```python
from build123d import *

# Parameters (mm, degrees)
PAD_DEPTH = 2.3


with BuildPart() as part:
    # Sketch → Pad (new body)
    with BuildSketch(Plane.XY):
        with BuildLine():
            Line((0, 0), (50, 0))
            Line((50, 0), (50, 30))
            Line((44.25, 30), (50, 30))
            Line((44.25, 30), (44.25, 23))
            ThreePointArc((39.75, 23), (42, 20.75), (44.25, 23))
            Line((39.75, 23), (39.75, 30))
            Line((39.75, 30), (34.25, 30))
            Line((34.25, 30), (34.25, 23))
            ThreePointArc((29.75, 23), (32, 20.75), (34.25, 23))
            Line((29.75, 23), (29.75, 30))
            Line((29.75, 30), (20.25, 30))
            Line((20.25, 30), (20.25, 23))
            ThreePointArc((15.75, 23), (18, 20.75), (20.25, 23))
            Line((15.75, 23), (15.75, 30))
            Line((15.75, 30), (10.25, 30))
            Line((10.25, 30), (10.25, 23))
            ThreePointArc((5.75, 23), (8, 20.75), (10.25, 23))
            Line((5.75, 23), (5.75, 30))
            Line((5.75, 30), (0, 30))
            Line((0, 30), (0, 0))
        make_face()
    extrude(amount=PAD_DEPTH)


solid = part.part
```
Input: part model. Units: mm. Frame: model coordinates. A direction names the side the tool comes from. Coordinates: 2 decimals unless noted, no trailing zeros. Write each loop counter-clockwise with the first axis right and the second up, starting at its lowest first coordinate (ties: lowest second). Pieces come first, ordered by that corner, then holes. Notation, with made-up numbers: (-5, -36) -> (42, -36) arc R31 cw to (42, -9) -> close; hole circle Ø1 at (75, 61). An arc over 180 degrees is marked (long way). Answer as a JSON object with one key per item and string values.
1. Material intervals for line 1 (X direction, y = 28.25, z = 1.2); line 2 (Y direction, x = 33.5, z = 1.45); line 3 (Y direction, x = 7, z = 1.3), sorted ascending. Write a range as from..to.
Result set:
{"line 1": "x = 0..5.75, 10.25..15.75, 20.25..29.75, 34.25..39.75, 44.25..50", "line 2": "y = 0..21.32", "line 3": "y = 0..20.98"}
2. Section C-C on x = 42. Return the cut outline in (y, z), then the cut area to 3 significant figures.
Result set:
{"outline": "(0, 0) -> (20.75, 0) -> (20.75, 2.3) -> (0, 2.3) -> close", "area": "47.7 mm2"}
3. Access query for faces 4 (the face through (25, 0, 1)), 5 (the face through (15.75, 26, 1)). Directions: +Z, -Z, +X, -X, +Y, -Y. A direction counts if a zero-diameter tool reaches every point of the face in a straight line with its end or side. Return the directions, or none.
Result set:
{"face 4": "+Z, -Z, +X, -X, -Y", "face 5": "+Z, -Z, +Y"}
4. Mould query, pull axis X, two halves, no side actions, for faces 1 (the face through (7.95, 20.75, 1.13)), 2 (the face through (0, 15, 1)), 3 (the face through (47, 30, 1)). Classes: released by +X, released by -X, zero draft, split by the parting line, or undercut.
Result set:
{"face 1": "undercut", "face 2": "released by -X", "face 3": "zero draft"}
5. Section B-B on z = 1.2. Return the cut outline in (x, y).
Result set:
{"outline": "(0, 0) -> (50, 0) -> (50, 30) -> (44.25, 30) -> (44.25, 23) arc R2.25 cw to (39.75, 23) -> (39.75, 30) -> (34.25, 30) -> (34.25, 23) arc R2.25 cw to (29.75, 23) -> (29.75, 30) -> (20.25, 30) -> (20.25, 23) arc R2.25 cw to (15.75, 23) -> (15.75, 30) -> (10.25, 30) -> (10.25, 23) arc R2.25 cw to (5.75, 23) -> (5.75, 30) -> (0, 30) -> close"}
6. Section A-A on y = 27.5. Return the cut outline in (x, z).
Result set:
{"outline": "(0, 0) -> (5.75, 0) -> (5.75, 2.3) -> (0, 2.3) -> close; (10.25, 0) -> (15.75, 0) -> (15.75, 2.3) -> (10.25, 2.3) -> close; (20.25, 0) -> (29.75, 0) -> (29.75, 2.3) -> (20.25, 2.3) -> close; (34.25, 0) -> (39.75, 0) -> (39.75, 2.3) -> (34.25, 2.3) -> close; (44.25, 0) -> (50, 0) -> (50, 2.3) -> (44.25, 2.3) -> close"}
